Geometry check sheet. Reference: the model listing, model coordinates, mm. Give positions to 0.01 mm unless a question says otherwise; leave off trailing zeros. Write each loop counter-clockwise with the first axis right and the second up, starting at its lowest first coordinate (ties: lowest second). Pieces come first, ordered by that corner, then holes. Notation, with made-up numbers: (86, 10) - (116, 10) arc R12 cw to (116, 24) - close; hole circle Ø7 at (-36.75, 2.5). An arc over 180 degrees is marked (long way). Write item = value, one per line. Start each with the question number.
(1) Section check C-C, the plane y = -12.7. Give the number of separate pieces and of enclosed holes in the cut face, plus the area to 3 significant figures.
(2) Thickness scan on L1, parallel to Y at x = 25.4, z = 0.85; L2, parallel to Y at x = 63.5, z = 0.7; L3, parallel to X at y = 17.5, z = -0.7. Record the ranges inside material, lowest first.
(3) Depth check by flat-ended pin: pin 1 Ø1.6 at (y, z) = (24, 0) entering from -X; pin 2 Ø1.5 at (x, z) = (86, 1) entering from +Y; pin 3 Ø1 at (y, z) = (34, 0.5) entering from +X; pin 4 Ø4 at (x, y) = (12.7, -25.4) entering from +Z. Enter the tip coordinate at first touch or a pass-through.
(4) Section check D-D, the plane x = 50.8. Enter the section's corners in (y, z).
(5) Section check B-B, the plane y = 38.1. Enter the section's corners in (x, z).
(6) Section check A-A, the plane x = 88.9. Enter the section's corners in (y, z), plus the area to 3 significant figures.
```python
from build123d import *

# Parameters (mm, degrees)
SKETCH1_W           = 101.6
SKETCH1_H           = 50.8
SKETCH1_R           = 2.4892
SKETCH1_W_2         = 25.4
BOSS_EXTRUDE1_DEPTH = 1.5875
FILLET1_R           = 5.08


with BuildPart() as part:
    # Sketch1 → Boss-Extrude1 (new, symmetric)
    # profile 1 of 2: a face of its own
    with BuildSketch(Plane.XY):
        with Locations((50.8, -25.4)):
            Rectangle(SKETCH1_W, SKETCH1_H)
        with Locations((12.7, -12.7)):
            Circle(SKETCH1_R, mode=Mode.SUBTRACT)
        with Locations((12.7, -25.4)):
            Circle(SKETCH1_R, mode=Mode.SUBTRACT)
        with Locations((88.9, -12.7)):
            Circle(SKETCH1_R, mode=Mode.SUBTRACT)
        with Locations((76.2, -12.7)):
            Circle(SKETCH1_R, mode=Mode.SUBTRACT)
        with Locations((63.5, -12.7)):
            Circle(SKETCH1_R, mode=Mode.SUBTRACT)
        with Locations((50.8, -12.7)):
            Circle(SKETCH1_R, mode=Mode.SUBTRACT)
        with Locations((38.1, -12.7)):
            Circle(SKETCH1_R, mode=Mode.SUBTRACT)
        with Locations((25.4, -12.7)):
            Circle(SKETCH1_R, mode=Mode.SUBTRACT)
        with Locations((88.9, -25.4)):
            Circle(SKETCH1_R, mode=Mode.SUBTRACT)
        with Locations((76.2, -25.4)):
            Circle(SKETCH1_R, mode=Mode.SUBTRACT)
        with Locations((63.5, -25.4)):
            Circle(SKETCH1_R, mode=Mode.SUBTRACT)
        with Locations((50.8, -25.4)):
            Circle(SKETCH1_R, mode=Mode.SUBTRACT)
        with Locations((38.1, -25.4)):
            Circle(SKETCH1_R, mode=Mode.SUBTRACT)
        with Locations((25.4, -25.4)):
            Circle(SKETCH1_R, mode=Mode.SUBTRACT)
        with Locations((88.9, -38.1)):
            Circle(SKETCH1_R, mode=Mode.SUBTRACT)
        with Locations((76.2, -38.1)):
            Circle(SKETCH1_R, mode=Mode.SUBTRACT)
        with Locations((63.5, -38.1)):
            Circle(SKETCH1_R, mode=Mode.SUBTRACT)
        with Locations((50.8, -38.1)):
            Circle(SKETCH1_R, mode=Mode.SUBTRACT)
        with Locations((38.1, -38.1)):
            Circle(SKETCH1_R, mode=Mode.SUBTRACT)
        with Locations((25.4, -38.1)):
            Circle(SKETCH1_R, mode=Mode.SUBTRACT)
        with Locations((12.7, -38.1)):
            Circle(SKETCH1_R, mode=Mode.SUBTRACT)
    # profile 2 of 2: a face of its own
    with BuildSketch(Plane.XY):
        with Locations((56.6928, 25.4)):
            Rectangle(SKETCH1_W_2, SKETCH1_H)
        with Locations((56.6928, 12.7)):
            Circle(SKETCH1_R, mode=Mode.SUBTRACT)
        with Locations((56.6928, 25.4)):
            Circle(SKETCH1_R, mode=Mode.SUBTRACT)
        with Locations((56.6928, 38.1)):
            Circle(SKETCH1_R, mode=Mode.SUBTRACT)
    extrude(amount=BOSS_EXTRUDE1_DEPTH, both=True)

    # Fillet1
    fillet1_edges = [part.edges().sort_by_distance(p)[0] for p in [
        (101.6, -50.8, 0),
        (0, -50.8, 0),
        (0, 0, 0),
        (43.9928, 0, 0),
        (43.9928, 50.8, 0),
        (69.3928, 50.8, 0),
        (69.3928, 0, 0),
        (101.6, 0, 0),
    ]]
    fillet(fillet1_edges, radius=FILLET1_R)


solid = part.part
```
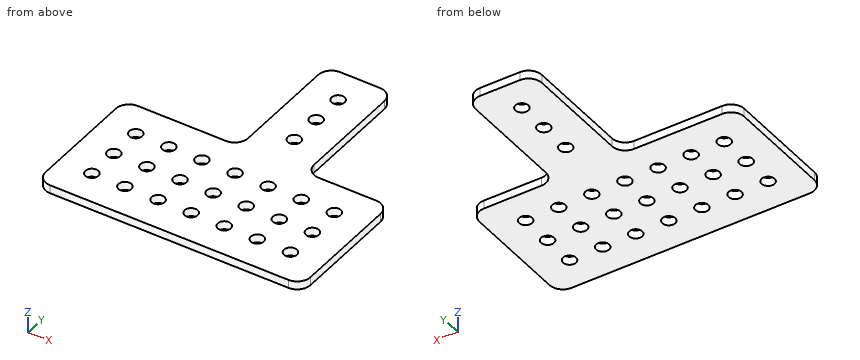
Model answer:
q1.separate_pieces = 8
q1.enclosed_holes = 0
q1.area = 212 mm²
q2.L1 = -50.8 to -40.59, -35.61 to -27.89, -22.91 to -15.19, -10.21 to 0
q2.L2 = -50.8 to -40.59, -35.61 to -27.89, -22.91 to -15.19, -10.21 to 50.8
q2.L3 = 43.99 to 69.39
q3.pin_1 = 43.99
q3.pin_2 = 0
q3.pin_3 = 69.39
q3.pin_4 = through
q4.outline = (-50.8, -1.59) - (-40.59, -1.59) - (-40.59, 1.59) - (-50.8, 1.59) - close; (-35.61, -1.59) - (-27.89, -1.59) - (-27.89, 1.59) - (-35.61, 1.59) - close; (-22.91, -1.59) - (-15.19, -1.59) - (-15.19, 1.59) - (-22.91, 1.59) - close; (-10.21, -1.59) - (50.8, -1.59) - (50.8, 1.59) - (-10.21, 1.59) - close
q5.outline = (43.99, -1.59) - (54.2, -1.59) - (54.2, 1.59) - (43.99, 1.59) - close; (59.18, -1.59) - (69.39, -1.59) - (69.39, 1.59) - (59.18, 1.59) - close
q6.outline = (-50.8, -1.59) - (-40.59, -1.59) - (-40.59, 1.59) - (-50.8, 1.59) - close; (-35.61, -1.59) - (-27.89, -1.59) - (-27.89, 1.59) - (-35.61, 1.59) - close; (-22.91, -1.59) - (-15.19, -1.59) - (-15.19, 1.59) - (-22.91, 1.59) - close; (-10.21, -1.59) - (0, -1.59) - (0, 1.59) - (-10.21, 1.59) - close
q6.area = 114 mm²
